```python
from build123d import *

# Parameters (mm, degrees)
F1_DEPTH = 6
F2_R     = 3.54
F3_DEPTH = 2.65
F4_R     = 2.5
F5_DEPTH = 25
F6_R     = 2


with BuildPart() as f1:
    # F0 (on Top) → F1 (new body)
    with BuildSketch(Plane.XY):
        Polygon((2.6685, -5.054613), (5.711673, -0.216318), (3.043173, 4.838295), (-2.6685, 5.054613), (-5.711673, 0.216318), (-3.043173, -4.838295), align=None)
    extrude(amount=F1_DEPTH)

    # F2 (on face) → F3 (join)
    with BuildSketch(Plane.XY.offset(6)):
        Circle(F2_R)
    extrude(amount=F3_DEPTH)

    # F4 (on face) → F5 (cut)
    with BuildSketch(Plane.XY.offset(8.65)):
        Circle(F4_R)
    extrude(amount=-F5_DEPTH, mode=Mode.SUBTRACT)

    # F6
    f6_edges = [f1.edges().sort_by_distance(p)[0] for p in [
        (2.6685, -5.054613, 3),
        (5.711673, -0.216318, 3),
        (-3.043173, -4.838295, 3),
        (-5.711673, 0.216318, 3),
        (-2.6685, 5.054613, 3),
        (3.043173, 4.838295, 3),
    ]]
    fillet(f6_edges, radius=F6_R)


solid = f1.part
```
Geometry check sheet. Reference: the model listing, model coordinates, mm. A direction names the side the tool comes from. Give positions to 0.01 mm unless a question says otherwise; leave off trailing zeros. Loops run counter-clockwise (first coordinate to the right, second up) from the corner with the lowest first, then second, coordinate; pieces in that order, holes last. Notation, with made-up numbers: M 45,72 L 74,72 A33 cw 74,102 Z; hole C 21,-18.75 d1. An arc over 180 degrees is marked long. Write item = value, one per line. Start each with the question number.
1. Section check D-D, the plane z = 8. Enter the section's corners in (x, y).
2. Thickness scan on probe 1 along X at (y, z) = (-2, 4.5); probe 2 along Z at (x, y) = (1.5, 4); probe 3 along Y at (x, z) = (0, 0.75). Record the ranges inside material, lowest first.
3. Section check C-C, the plane y = 0. Enter the section's corners in (x, z), plus the area to 3 significant figures.
4. Draft check along Y on faces 1 (the face through (4.177, -2.656, 2.958)), 2 (the face through (-2.5, 1.2, 0)), 3 (the face through (-0.54, -2.44, 4.39)). Enter one of: +Y half, -Y half, draft (parallel to the pull), parting line (faces both ways), or undercut.
5. Section check A-A, the plane x = 0. Enter the section's corners in (y, z).
6. Tool access check on faces 4 (the face through (2, -2, 8.65)), 5 (the face through (3.377, 1.063, 7.306)). Record the directions out of +Z, -Z, +X, -X, +Y, -Y that give a thin tool (end or side, any length) a straight path to the whole face; none if there is none.
7. Section check B-B, the plane z = 1.5. Enter the section's corners in (x, y).
8. Go/stop test with flat-tipped pins: P1, Ø1.5, axis at y = -3, z = 6.5, coming from the -X side; P2, Ø3, axis at x = -2.5, z = 6.5, coming from the -Y side; P3, Ø2, axis at x = 4, z = 4.5, coming from the +Y side. Record where each tip stops, or that it passes through.
Values follow:
q1.outline = C 0,0 d7.08; hole C 0,0 d5
q2.probe_1 = -4.54 to -1.5, 1.5 to 4.59
q2.probe_2 = 0 to 6
q2.probe_3 = -4.95 to -2.5, 2.5 to 4.95
q3.outline = M -5.4,0 L -2.5,0 L -2.5,8.65 L -3.54,8.65 L -3.54,6 L -5.4,6 Z; M 2.5,0 L 5.4,0 L 5.4,6 L 3.54,6 L 3.54,8.65 L 2.5,8.65 Z
q3.area = 40.3 mm^2
q4.face_1 = -Y half
q4.face_2 = draft
q4.face_3 = undercut
q5.outline = M -4.95,0 L -2.5,0 L -2.5,8.65 L -3.54,8.65 L -3.54,6 L -4.95,6 Z; M 2.5,0 L 4.95,0 L 4.95,6 L 3.54,6 L 3.54,8.65 L 2.5,8.65 Z
q6.face_4 = +Z, +X, -X, +Y, -Y
q6.face_5 = +Z
q7.outline = M -5.17,-0.8 L -3.58,-3.82 A2 ccw -1.89,-4.88 L 1.51,-5.01 A2 ccw 3.28,-4.08 L 5.1,-1.19 A2 ccw 5.17,0.8 L 3.58,3.82 A2 ccw 1.89,4.88 L -1.51,5.01 A2 ccw -3.28,4.08 L -5.1,1.19 A2 ccw Z; hole C 0,0 d5
q8.P1 = -4.31
q8.P2 = -4.91
q8.P3 = 4.49
